Geometry: final body of the model. Coordinates: model frame, mm. A direction names the side the tool comes from. Give positions to 0.01 mm unless a question says otherwise; leave off trailing zeros. Order: outer loops, then holes, each group sorted by start corner. A loop starts at its lowest first (then second) coordinate and runs counter-clockwise, first axis right, second up. Notation, with made-up numbers: (65.5, -24) - (119.5, -24) arc R18 cw to (119.5, 8) - close; hole circle Ø2 at (34, 42.5). An arc over 180 degrees is marked (long way). Put each result on its own line as item: value. Start each with the question number.
1. Mould query, pull axis Y, two halves, no side actions, for faces 3 (the conical face through (9.49, 6.27, -5.75)), 4 (the flat face through (9, 25, 0)), 5 (the cylindrical face through (9.481, 50.438, -0.382)). Classes: pulls with the +Y half, pulls with the -Y half, needs draft (parallel to the pull), parting line crosses it, or undercut.
2. Ray query, line 1 along Y through (x, z) = (8.5, -2); line 2 along Y through (x, z) = (6.5, -4.5); line 3 along Y through (x, z) = (11.75, -2.5). Return the intervals inside material, ascending. Write a range as from..to.
3. First-contact query: P1, Ø7.5, axis at x = 9.525, y = 18.034, coming from the -Z side; P2, Ø4.5, axis at x = 9.52, y = 46.04, coming from the +Z side; P3, Ø3, axis at x = 17, z = -2.5, coming from the -Y side; P4, Ø1.5, axis at x = 5, z = -4.5, coming from the -Y side. Flat tips, straight axial feed; report the tip coordinate or a pass-through.
4. Section B-B on z = -4. Count the separate pieces of the cut face and the enclosed holes in it, plus the area to 3 significant figures.
5. Section A-A on y = 20.5. Return the cut outline in (x, z), plus the area to 3 significant figures.
6. Set-up query: faces 1 (the flat face through (9, 25, -6.35)), 2 (the cylindrical face through (12.933, 34.411, -1.728)). Return all of +Z, -Z, +X, -X, +Y, -Y with unobstructed straight access to the full face (end or side cutting, diameter ignored); none if empty.
from build123d import *

# Parameters (mm, degrees)
SKETCH1_W                                      = 6.35
SKETCH1_H                                      = 50.8
BODY_DEPTH                                     = 19.05
SKETCH2_R                                      = 5.207
PITCH_AXLE_OPENING_DEPTH                       = 6.35
CBORE_FOR_6_SOCKET_HEAD_CAP_SCREW1_D           = 3.7973
CBORE_FOR_6_SOCKET_HEAD_CAP_SCREW1_CBORE_D     = 7.14502
CBORE_FOR_6_SOCKET_HEAD_CAP_SCREW1_CBORE_DEPTH = 3.5052
F_6_32_TAPPED_HOLE1_D                          = 2.7051
F_6_32_TAPPED_HOLE1_DEPTH                      = 5.08
F_6_32_TAPPED_HOLE1_TIP                        = 0.81269403
SKETCH2_3_R                                    = 6.35
SKETCH2_3_R_2                                  = 5.207
PITCH_BEARING_RECESS_DEPTH                     = 3.96748
FILLET1_R                                      = 6.35
FILLET2_R                                      = 1.27


with BuildPart() as part:
    # Sketch1 → Body (new body)
    with BuildSketch(Plane(origin=(0, 0, 0), x_dir=(0, 0, -1), z_dir=(1, 0, 0))):
        with Locations((3.175, 25.4)):
            Rectangle(SKETCH1_W, SKETCH1_H)
    extrude(amount=BODY_DEPTH)

    # Sketch2 → Pitch Axle Opening (cut)
    with BuildSketch(Plane(origin=(0, 0, -6.35), x_dir=(-1, 0, 0), z_dir=(0, 0, -1))):
        with Locations((-9.525, 18.034)):
            Circle(SKETCH2_R)
    extrude(amount=-PITCH_AXLE_OPENING_DEPTH, mode=Mode.SUBTRACT)

    # CBORE for #6 Socket Head Cap Screw1 (through all)
    with Locations(Plane.XY):
        with Locations((9.525, 46.0375), (9.525, 33.3375)):
            CounterBoreHole(CBORE_FOR_6_SOCKET_HEAD_CAP_SCREW1_D / 2, CBORE_FOR_6_SOCKET_HEAD_CAP_SCREW1_CBORE_D / 2, CBORE_FOR_6_SOCKET_HEAD_CAP_SCREW1_CBORE_DEPTH)

    # #6-32 Tapped Hole1
    with Locations(Plane(origin=(9.525, 6.034, 0), x_dir=(1, 0, 0), z_dir=(0, 0, 1))):
        with Locations((0, 0)):
            Hole(F_6_32_TAPPED_HOLE1_D / 2, depth=F_6_32_TAPPED_HOLE1_DEPTH)
            with Locations((0, 0, -(F_6_32_TAPPED_HOLE1_DEPTH + F_6_32_TAPPED_HOLE1_TIP / 2))):  # 118° drill point
                Cone(0, F_6_32_TAPPED_HOLE1_D / 2, F_6_32_TAPPED_HOLE1_TIP, mode=Mode.SUBTRACT)

    # Sketch2<3> → Pitch Bearing Recess (cut)
    with BuildSketch(Plane(origin=(0, 0, -6.35), x_dir=(-1, 0, 0), z_dir=(0, 0, -1))):
        with Locations((-9.525, 18.034)):
            Circle(SKETCH2_3_R)
        with Locations((-9.525, 18.034)):
            Circle(SKETCH2_3_R_2, mode=Mode.SUBTRACT)
    extrude(amount=-PITCH_BEARING_RECESS_DEPTH, mode=Mode.SUBTRACT)

    # Fillet1
    fillet1_edges = [part.edges().sort_by_distance(p)[0] for p in [
        (19.05, 50.8, -3.175),
        (19.05, 0, -3.175),
        (0, 50.8, -3.175),
        (0, 0, -3.175),
    ]]
    fillet(fillet1_edges, radius=FILLET1_R)

    # Fillet2
    # the kernel refuses this fillet: 1.27 mm, written as the material it takes off along each edge
    with BuildSketch(Plane(origin=(6.35, 50.8, 0), x_dir=(0, -1, 0), z_dir=(1, 0, 0))) as fillet2_piece_1:
        with BuildLine():
            CenterArc((FILLET2_R, FILLET2_R), FILLET2_R, 180, 90)
            Line((0, FILLET2_R), (0, 0))
            Line((0, 0), (FILLET2_R, 0))
        make_face()
    extrude(amount=6.35, mode=Mode.SUBTRACT)
    with BuildSketch(Plane(origin=(0, 6.35, 0), x_dir=(1, 0, 0), z_dir=(0, 1, 0))) as fillet2_piece_2:
        with BuildLine():
            CenterArc((FILLET2_R, FILLET2_R), FILLET2_R, 180, 90)
            Line((0, FILLET2_R), (0, 0))
            Line((0, 0), (FILLET2_R, 0))
        make_face()
    extrude(amount=38.1, mode=Mode.SUBTRACT)
    with BuildSketch(Plane(origin=(6.35, 0, 0), x_dir=(0, 1, 0), z_dir=(1, 0, 0))) as fillet2_piece_3:
        with BuildLine():
            CenterArc((FILLET2_R, -FILLET2_R), FILLET2_R, 90, 90)
            Line((0, -FILLET2_R), (0, 0))
            Line((0, 0), (FILLET2_R, 0))
        make_face()
    extrude(amount=6.35, mode=Mode.SUBTRACT)
    with BuildSketch(Plane(origin=(19.05, 6.35, 0), x_dir=(-1, 0, 0), z_dir=(0, 1, 0))) as fillet2_piece_4:
        with BuildLine():
            CenterArc((FILLET2_R, -FILLET2_R), FILLET2_R, 90, 90)
            Line((0, -FILLET2_R), (0, 0))
            Line((0, 0), (FILLET2_R, 0))
        make_face()
    extrude(amount=38.1, mode=Mode.SUBTRACT)
    with BuildSketch(Plane(origin=(12.7, 6.35, 0), x_dir=(0, -1, 0), z_dir=(-1, 0, 0))) as fillet2_piece_5:
        with BuildLine():
            CenterArc((6.35 - FILLET2_R, -FILLET2_R), FILLET2_R, 0, 90)
            Line((6.35, -FILLET2_R), (6.35, 0))
            Line((6.35, 0), (6.35 - FILLET2_R, 0))
        make_face()
    revolve(axis=Axis((12.7, 6.35, 0), (0, 0, 1)), revolution_arc=90, mode=Mode.SUBTRACT)
    with BuildSketch(Plane(origin=(6.35, 6.35, 0), x_dir=(0, -1, 0), z_dir=(1, 0, 0))) as fillet2_piece_6:
        with BuildLine():
            CenterArc((6.35 - FILLET2_R, FILLET2_R), FILLET2_R, 270, 90)
            Line((6.35, FILLET2_R), (6.35, 0))
            Line((6.35, 0), (6.35 - FILLET2_R, 0))
        make_face()
    revolve(axis=Axis((6.35, 6.35, 0), (0, 0, -1)), revolution_arc=90, mode=Mode.SUBTRACT)
    with BuildSketch(Plane(origin=(12.7, 44.45, 0), x_dir=(1, 0, 0), z_dir=(0, -1, 0))) as fillet2_piece_7:
        with BuildLine():
            CenterArc((6.35 - FILLET2_R, -FILLET2_R), FILLET2_R, 0, 90)
            Line((6.35, -FILLET2_R), (6.35, 0))
            Line((6.35, 0), (6.35 - FILLET2_R, 0))
        make_face()
    revolve(axis=Axis((12.7, 44.45, 0), (0, 0, 1)), revolution_arc=90, mode=Mode.SUBTRACT)
    with BuildSketch(Plane(origin=(6.35, 44.45, 0), x_dir=(-1, 0, 0), z_dir=(0, -1, 0))) as fillet2_piece_8:
        with BuildLine():
            CenterArc((6.35 - FILLET2_R, FILLET2_R), FILLET2_R, 270, 90)
            Line((6.35, FILLET2_R), (6.35, 0))
            Line((6.35, 0), (6.35 - FILLET2_R, 0))
        make_face()
    revolve(axis=Axis((6.35, 44.45, 0), (0, 0, -1)), revolution_arc=90, mode=Mode.SUBTRACT)


solid = part.part
Resolved:
1. face 3: undercut
1. face 4: needs draft
1. face 5: pulls with the +Y half
2. line 1: 0..5.15, 6.92..12.93, 23.14..29.92, 36.76..42.62, 49.46..50.8
2. line 2: 0..12.45, 23.62..50.8
2. line 3: 0..12.09, 23.98..30.54, 36.13..43.24, 48.83..50.8
3. P1: through
3. P2: z = -3.51
3. P3: y = 0.65
3. P4: y = 0.03
4. separate pieces: 1
4. enclosed holes: 4
4. area: 778 mm^2
5. outline: (0, -6.35) - (3.67, -6.35) - (3.67, -2.38) - (4.94, -2.38) - (4.94, 0) - (1.27, 0) arc R1.27 ccw to (0, -1.27) - close; (14.11, -2.38) - (15.38, -2.38) - (15.38, -6.35) - (19.05, -6.35) - (19.05, -1.27) arc R1.27 ccw to (17.78, 0) - (14.11, 0) - close
5. area: 52.0 mm^2
6. face 1: -Z, +X, -X, +Y, -Y
6. face 2: +Z
